```python
from build123d import *

# Parameters (mm, degrees)
F2_W     = 50.8
F2_H     = 50.8
F3_DEPTH = 12.7
F4_W     = 38.1
F4_H     = 12.7
F5_DEPTH = 25.4


with BuildPart() as f1:
    # F0 (on Front) → F1 (revolve)
    with BuildSketch(Plane.XZ):
        with BuildLine():
            Line((0, 12.7), (0, -12.7))
            add(Edge.make_bspline(
                [(0, -12.7), (31.75, -12.7), (31.75, 0), (31.75, 12.7), (0, 12.7)],
                knots=[1.5707963268, 1.5707963268, 1.5707963268, 3.1415926536, 3.1415926536, 4.7123889804, 4.7123889804, 4.7123889804], degree=2, weights=[1, 0.7071067812, 1, 0.7071067812, 1]))
        make_face()
    revolve(axis=Axis((0, 0, 0), (0, 0, -1)))

    # F2 (on Top) → F3 (cut, symmetric)
    with BuildSketch(Plane.XY):
        with Locations((0, -12.7)):
            Rectangle(F2_W, F2_H)
    extrude(amount=F3_DEPTH, both=True, mode=Mode.SUBTRACT)

    # F4 (on face) → F5 (cut)
    with BuildSketch(Plane.XZ.offset(-12.7)):
        Rectangle(F4_W, F4_H)
    extrude(amount=-F5_DEPTH, mode=Mode.SUBTRACT)


solid = f1.part
```
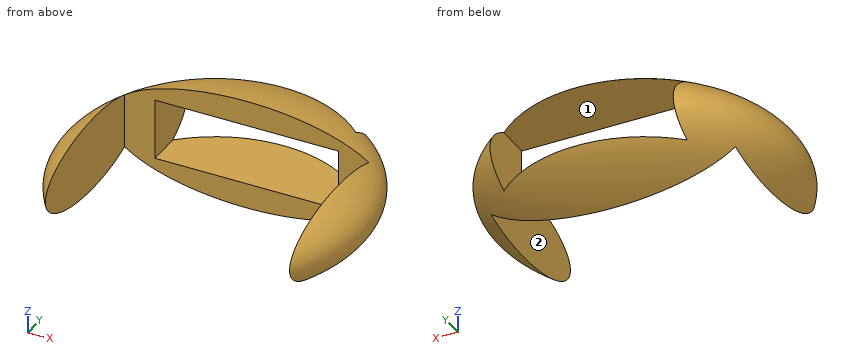
Check sheet for the modelled part. Datum: model origin and axes. Units: mm. Face numbers are marked on the shaded views. A direction names the side the tool comes from. Round coordinates to 2 decimals unless told otherwise and drop trailing zeros. Answer as a JSON object with one key per item and string values.
1. Section check A-A (y = 21). State how many separate pieces and enclosed holes the cut face has, plus the area to 3 significant figures.
Reply:
{"separate pieces": "4", "enclosed holes": "0", "area": "230 mm²"}
2. Gauge pin test, flat ends, axial feed: P1, Ø12, axis at y = -3.5, z = 8.5, coming from the -X side; P2, Ø1, axis at y = 5.5, z = 6, coming from the -X side; P3, Ø3, axis at x = -3, y = 13.5, coming from the +Z side; P4, Ø12, axis at x = 9.5, y = 4.5, coming from the -Z side. Record the tip position at first contact, or that the pin passes through.
Reply:
{"P1": "stops at x = -30.99", "P2": "stops at x = -28.09", "P3": "stops at z = 11.62", "P4": "passes through"}
3. Scan lines: line 1 (X direction, y = 19, z = 2); line 2 (X direction, y = 2, z = 5.5); line 3 (Z direction, x = -0.5, y = 14). Record each from-to range of solid material in increasing order.
Reply:
{"line 1": "x = -24.94 to -19.05, 19.05 to 24.94", "line 2": "x = -28.55 to -25.4, 25.4 to 28.55", "line 3": "z = -11.4 to -6.35, 6.35 to 11.4"}
4. Access from +Z, -Z, +X, -X, +Y, -Y to the whole of each face (thin tool, end or side, straight path). Record for the marked faces 1 and 2.
Reply:
{"face 1": "+Y, -Y", "face 2": "+Z, -Z, -Y"}
